from build123d import *

# Parameters (mm, degrees)
F1_DEPTH      = 0.381
F1_DEPTH_BACK = 0.381
F2_R          = 1.908991
F3_DEPTH      = 1.27
F3_DEPTH_BACK = 0.6858
F4_DEPTH      = 0.9398
F4_DEPTH_BACK = 1.8034


with BuildPart() as f1:
    # F0 (on Top) → F1 (new body, two sides)
    with BuildSketch(Plane.XY) as f1_sk:
        with BuildLine():
            Line((19.605453, 3.353871), (-19.605453, 3.353871))
            ThreePointArc((-19.605453, 3.353871), (-21.346986, 2.632504), (-22.068353, 0.89097))
            Line((-22.068353, 0.89097), (-22.068353, -0.89097))
            ThreePointArc((-22.068353, -0.89097), (-21.346986, -2.632504), (-19.605453, -3.353871))
            Line((-19.605453, -3.353871), (19.605453, -3.353871))
            ThreePointArc((19.605453, -3.353871), (21.346986, -2.632504), (22.068353, -0.89097))
            Line((22.068353, -0.89097), (22.068353, 0.89097))
            ThreePointArc((22.068353, 0.89097), (21.346986, 2.632504), (19.605453, 3.353871))
        make_face()
    extrude(amount=F1_DEPTH)
    extrude(f1_sk.sketch, amount=-F1_DEPTH_BACK)

    # F2 (on face) → F3 (cut, two sides)
    with BuildSketch(Plane.XY.offset(0.381)) as f3_sk:
        with Locations((-19.042145, 0)):
            Circle(F2_R)
    extrude(amount=-F3_DEPTH, mode=Mode.SUBTRACT)
    extrude(f3_sk.sketch, amount=-F3_DEPTH_BACK, mode=Mode.SUBTRACT)

    # F2 (on face) → F4 (cut, two sides)
    with BuildSketch(Plane.XY.offset(0.381)) as f4_sk:
        with Locations((19.042145, 0)):
            Circle(F2_R)
    extrude(amount=F4_DEPTH, mode=Mode.SUBTRACT)
    extrude(f4_sk.sketch, amount=-F4_DEPTH_BACK, mode=Mode.SUBTRACT)


solid = f1.part
Geometry: final body of the model. Coordinates: model frame, mm. Coordinates: 2 decimals unless noted, no trailing zeros. Loops run counter-clockwise (first coordinate to the right, second up) from the corner with the lowest first, then second, coordinate; pieces in that order, holes last. Notation, with made-up numbers: (-21, 42) - (30, 42) arc R27 cw to (30, 61) - close; hole circle Ø6 at (47.25, 79). An arc over 180 degrees is marked (long way). Put each result on its own line as item: value. Start each with the question number.
Q1. Cut plane B-B, the plane y = 0. Return loops of the section in (x, z), and give its area (3 significant figures).
Q2. Cut plane A-A, the plane z = -0.15. Return loops of the section in (x, y), and give its area (3 significant figures).
Q3. Line query: line 1 (X direction, y = 0.25, z = 0); line 2 (X direction, y = -0.75, z = -0.3); line 3 (X direction, y = 2.5, z = 0.3). Output: solid intervals per line, ascending.
Q4. Cut plane C-C, the plane x = -19. Return loops of the section in (y, z), and give its area (3 significant figures).
Q5. Pull-direction query (Y, two-part tool) for faces 1 (the cylindrical face through (-21.37, -2.61, 0.01)), 2 (the cylindrical face through (-17.28, -0.73, 0.01)), 3 (the flat face through (0, 0, -0.381)); classes: released by +Y, released by -Y, zero draft, split by the parting line, or undercut.
Filled sheet:
1. outline: (-22.07, -0.38) - (-20.95, -0.38) - (-20.95, 0.38) - (-22.07, 0.38) - close; (-17.13, -0.38) - (17.13, -0.38) - (17.13, 0.38) - (-17.13, 0.38) - close; (20.95, -0.38) - (22.07, -0.38) - (22.07, 0.38) - (20.95, 0.38) - close
1. area: 27.8 mm²
2. outline: (-22.07, -0.89) arc R2.46 ccw to (-19.61, -3.35) - (19.61, -3.35) arc R2.46 ccw to (22.07, -0.89) - (22.07, 0.89) arc R2.46 ccw to (19.61, 3.35) - (-19.61, 3.35) arc R2.46 ccw to (-22.07, 0.89) - close; hole circle Ø3.82 at (-19.04, 0); hole circle Ø3.82 at (19.04, 0)
2. area: 268 mm²
3. line 1: -22.07 to -20.93, -17.15 to 17.15, 20.93 to 22.07
3. line 2: -22.07 to -20.8, -17.29 to 17.29, 20.8 to 22.07
3. line 3: -21.47 to 21.47
4. outline: (-3.35, -0.38) - (-1.91, -0.38) - (-1.91, 0.38) - (-3.35, 0.38) - close; (1.91, -0.38) - (3.35, -0.38) - (3.35, 0.38) - (1.91, 0.38) - close
4. area: 2.20 mm²
5. face 1: released by -Y
5. face 2: undercut
5. face 3: zero draft
